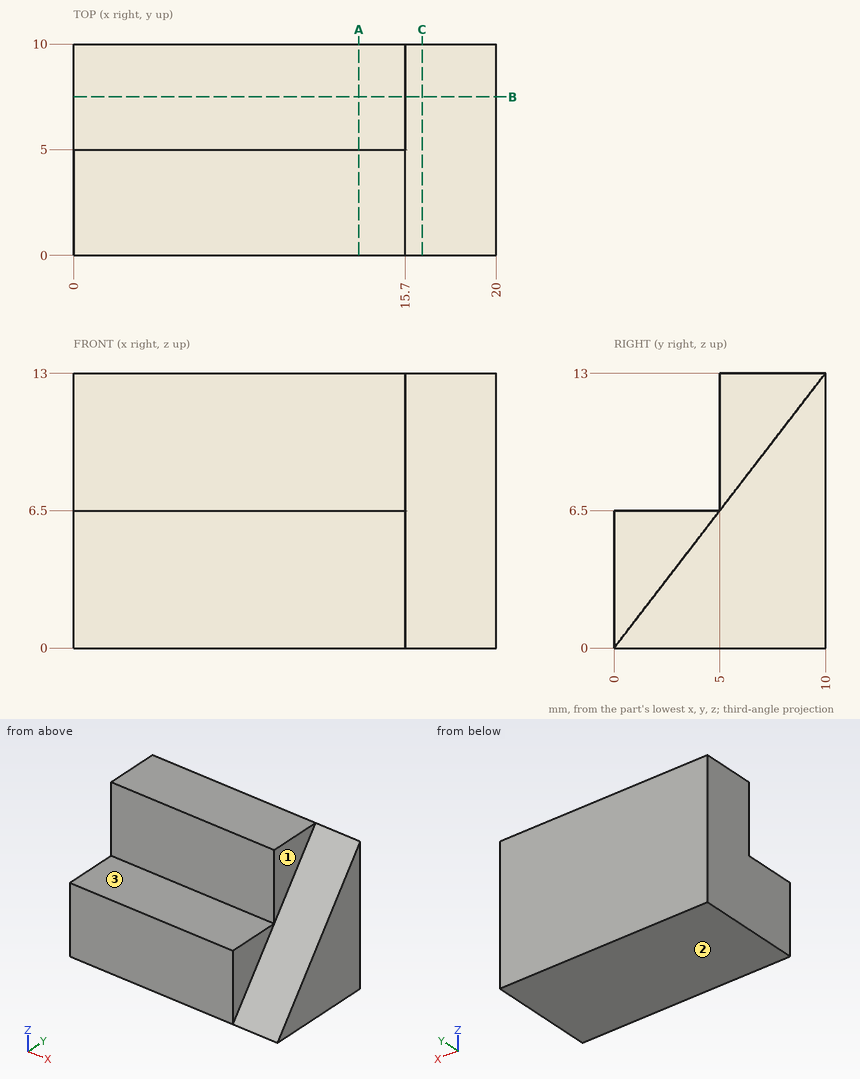
Can you work these out from the drawing? Everything is in mm from the part's minimum corner. A direction names the side the tool comes from. Give positions to 0.01 mm unless a question says otherwise; leave off trailing zeros. Loops run counter-clockwise (first coordinate to the right, second up) from the corner with the lowest first, then second, coordinate; pieces in that order, holes last. Notation, with made-up numbers: (-29.5, 80) -> (26.5, 80) arc R5 ccw to (26.5, 86) -> close; hole circle Ø1 at (-13.75, 43.5). An arc over 180 degrees is marked (long way). Put each result on its own line as item: value.
(1) Please list where these lines run through material, in increasing order: probe 1 along X at (y, z) = (0.75, 1.5); probe 2 along Y at (x, z) = (9.5, 8.75); probe 3 along Z at (x, y) = (11.75, 3). Write a range as [from, to].
Computed:
probe 1: [0, 15.7]
probe 2: [5, 10]
probe 3: [0, 6.5]
(2) Imagine slicing it at C-C on x = 16.5. Write out the boundary of the cut face in (y, z), plus the area to 3 significant figures.
Computed:
outline: (0, 0) -> (10, 0) -> (10, 13) -> close
area: 65.0 mm^2
(3) I'm going to push flat-ended pins straight in: pin 1 Ø2 at (y, z) = (3.5, 10) entering from -X; pin 2 Ø6 at (x, y) = (4, 1.5) entering from +Z; pin 3 Ø4 at (x, z) = (6.5, 11.5) entering from -Y. Where does each tip first touch, or does it pass through?
Computed:
pin 1: through
pin 2: z = 6.5
pin 3: y = 5
(4) Imagine slicing it at B-B on y = 7.5. Write out the boundary of the cut face in (x, z).
Computed:
outline: (0, 0) -> (20, 0) -> (20, 9.75) -> (15.7, 9.75) -> (15.7, 13) -> (0, 13) -> close
(5) For the marked faces 1, 2 and 3, which set-ups out of +Z, -Z, +X, -X, +Y, -Y let a thin tool reach every point of the face, with its end or its side?
Computed:
face 1: +Z, +X, -Y
face 2: -Z, +X, -X, +Y, -Y
face 3: +Z, +X, -X, -Y
(6) Imagine slicing it at A-A on x = 13.5. Write out the boundary of the cut face in (y, z).
Computed:
outline: (0, 0) -> (10, 0) -> (10, 13) -> (5, 13) -> (5, 6.5) -> (0, 6.5) -> close
